Check sheet for the modelled part. Datum: model origin and axes. Units: mm. Face numbers are marked on the shaded views. A direction names the side the tool comes from. Round coordinates to 2 decimals unless told otherwise and drop trailing zeros. Order: outer loops, then holes, each group sorted by start corner. A loop starts at its lowest first (then second) coordinate and runs counter-clockwise, first axis right, second up.
(1) Mould release check, pull along X, two halves, no side actions. Record for the marked faces 1, 2 and 3: released by +X, released by -X, zero draft, split by the parting line, or undercut.
(2) Depth check by flat-ended pin: pin 1 (1.5 mm diameter, centred on x = -23.5, y = -3, fed in from +Z); pin 2 (8 mm diameter, centred on x = 11, y = -14.5, fed in from -Z); pin 3 (3 mm diameter, centred on x = -17.5, y = -14.5, fed in from -Z). Enter the tip coordinate at first touch or a pass-through.
(3) Sectioned sample at C-C, the plane y = -4. Count the separate pieces of the cut face and the enclosed holes in it, and give its area (3 significant figures).
(4) Sectioned sample at B-B, the plane y = -12.5. Enter the section's corners in (x, z).
(5) Tool access check on the marked faces 4 and 5. Record the directions out of +Z, -Z, +X, -X, +Y, -Y that give a thin tool (end or side, any length) a straight path to the whole face; none if there is none.
(6) Thickness scan on probe 1 along Z at (x, y) = (0, -0.6); probe 2 along Z at (x, y) = (0, -9.5); probe 3 along X at (y, z) = (-2, -8). Record the ranges inside material, lowest first.
(7) Sectioned sample at A-A, the plane z = 0. Enter the section's corners in (x, y).
```python
from build123d import *

# Parameters (mm, degrees)
SKETCH_R        = 29.75
PAD_DEPTH       = 19
POCKET_DEPTH    = 2
SKETCH002_R     = 5
HOLE_DEPTH      = 17.001
SKETCH003_R     = 2.5
HOLE001_DEPTH   = 17.001
POCKET001_DEPTH = 7
SKETCH005_R     = 7
POCKET002_DEPTH = 2
FILLET_R        = 0.5


with BuildPart() as part:
    # Sketch → Pad (new body)
    with BuildSketch(Plane.XZ):
        Circle(SKETCH_R)
    extrude(amount=PAD_DEPTH)

    # Sketch001 (on Face3 of Pad) → Pocket (cut)
    with BuildSketch(Plane.XZ.offset(19)):
        Polygon((-10.2, 27.94678), (-10.2, 10.2), (-27.94678, 10.2), (-38.800591, 2.809986), (-27.94678, -10.2), (-10.2, -10.2), (-10.2, -27.94678), (0.437611, -41.292454), (10.2, -27.94678), (10.2, -10.2), (27.94678, -10.2), (40.756752, -1.838068), (27.94678, 10.2), (10.2, 10.2), (10.2, 27.94678), (-0.319049, 40.318684), align=None)
    extrude(amount=-POCKET_DEPTH, mode=Mode.SUBTRACT)

    # Sketch002 (on Face3 of Pocket) → Hole (cut, through all)
    with BuildSketch(Plane.XZ.offset(17)):
        Circle(SKETCH002_R)
    extrude(amount=-HOLE_DEPTH, mode=Mode.SUBTRACT)

    # Sketch003 (on Face3 of Hole) → Hole001 (cut, through all)
    with BuildSketch(Plane.XZ.offset(17)):
        with Locations((0, 22.5)):
            Circle(SKETCH003_R)
        with Locations((22.5, 0)):
            Circle(SKETCH003_R)
        with Locations((0, -22.5)):
            Circle(SKETCH003_R)
        with Locations((-22.5, 0)):
            Circle(SKETCH003_R)
    extrude(amount=-HOLE001_DEPTH, mode=Mode.SUBTRACT)

    # Sketch004 (on Face2 of Hole001) → Pocket001 (cut)
    with BuildSketch(Plane(origin=(0, 0, 0), x_dir=(1, 0, 0), z_dir=(0, 1, 0))):
        with BuildLine():
            ThreePointArc((-21.944444, -4.96904), (-15.909903, -15.909903), (-4.96904, -21.944444))
            ThreePointArc((-3.5, -18.929286), (-4.494881, -20.310013), (-4.96904, -21.944444))
            Line((-3.5, -8.831761), (-3.5, -18.929286))
            ThreePointArc((-8.831761, -3.5), (-6.717514, -6.717514), (-3.5, -8.831761))
            Line((-18.929286, -3.5), (-8.831761, -3.5))
            ThreePointArc((-21.944444, -4.96904), (-20.310013, -4.494881), (-18.929286, -3.5))
        make_face()
        with BuildLine():
            ThreePointArc((8.831761, 3.5), (6.717514, 6.717514), (3.5, 8.831761))
            Line((3.5, 18.929286), (3.5, 8.831761))
            ThreePointArc((3.5, 18.929286), (4.494881, 20.310013), (4.96904, 21.944444))
            ThreePointArc((21.944444, 4.96904), (15.909903, 15.909903), (4.96904, 21.944444))
            ThreePointArc((21.944444, 4.96904), (20.310013, 4.494881), (18.929286, 3.5))
            Line((8.831761, 3.5), (18.929286, 3.5))
        make_face()
        with BuildLine():
            ThreePointArc((18.929286, -3.5), (20.310013, -4.494881), (21.944444, -4.96904))
            ThreePointArc((4.96904, -21.944444), (15.909903, -15.909903), (21.944444, -4.96904))
            ThreePointArc((4.96904, -21.944444), (4.494881, -20.310013), (3.5, -18.929286))
            Line((3.5, -8.831761), (3.5, -18.929286))
            ThreePointArc((3.5, -8.831761), (6.717514, -6.717514), (8.831761, -3.5))
            Line((8.831761, -3.5), (18.929286, -3.5))
        make_face()
        with BuildLine():
            Line((-3.5, 8.831761), (-3.5, 18.929286))
            ThreePointArc((-4.96904, 21.944444), (-4.494881, 20.310013), (-3.5, 18.929286))
            ThreePointArc((-4.96904, 21.944444), (-15.909903, 15.909903), (-21.944444, 4.96904))
            ThreePointArc((-18.929286, 3.5), (-20.310013, 4.494881), (-21.944444, 4.96904))
            Line((-18.929286, 3.5), (-8.831761, 3.5))
            ThreePointArc((-3.5, 8.831761), (-6.717514, 6.717514), (-8.831761, 3.5))
        make_face()
    extrude(amount=-POCKET001_DEPTH, mode=Mode.SUBTRACT)

    # Sketch005 (on Face2 of Pocket001) → Pocket002 (cut)
    with BuildSketch(Plane(origin=(0, 0, 0), x_dir=(1, 0, 0), z_dir=(0, 1, 0))):
        Circle(SKETCH005_R)
    extrude(amount=-POCKET002_DEPTH, mode=Mode.SUBTRACT)

    # Sketch006 (on DatumPlane) → Groove (revolve, cut)
    with BuildSketch(Plane(origin=(29.75, 0, 0), x_dir=(-1, 0, 0), z_dir=(0, 0, -1))):
        Polygon((0, -14), (1.5, -19), (0, -19), align=None)
    revolve(axis=Axis((0, 0, 0), (0, 1, 0)), mode=Mode.SUBTRACT)

    # Fillet
    fillet_edges = [part.edges().sort_by_distance(p)[0] for p in [
        (-29.75, 0, 0),
    ]]
    fillet(fillet_edges, radius=FILLET_R)


solid = part.part
```
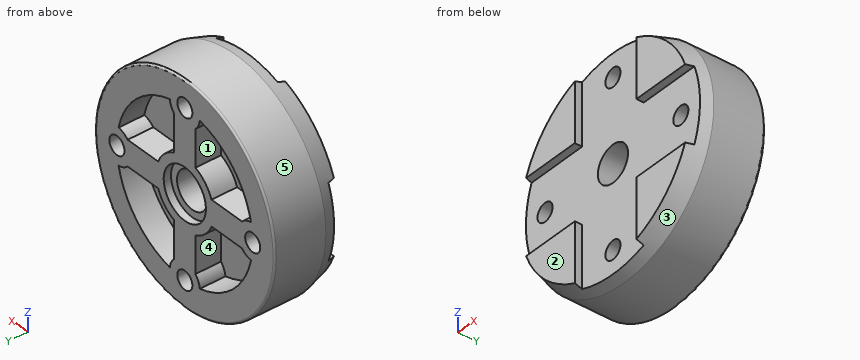
Derived:
1. face 1: undercut
1. face 2: zero draft
1. face 3: split by the parting line
2. pin 1: stops at z = 19.17
2. pin 2: stops at z = -28.91
2. pin 3: stops at z = -25.03
3. separate pieces: 1
3. enclosed holes: 9
3. area: 1,710 mm2
4. outline: circle Ø59.5 at (0, 0); hole circle Ø5 at (-22.5, 0); hole circle Ø10 at (0, 0); hole circle Ø5 at (0, -22.5); hole circle Ø5 at (0, 22.5); hole circle Ø5 at (22.5, 0)
5. face 4: +Y
5. face 5: +Y, -Y
6. probe 1: z = -29.75 to -25, -20 to -7, 7 to 20, 25 to 29.75
6. probe 2: z = -29.75 to -25, -20 to -5, 5 to 20, 25 to 29.75
6. probe 3: x = -28.65 to -21.03, -5.12 to 5.12, 21.03 to 28.65
7. outline: (-29.75, -14) - (-28.85, -17) - (-25, -17) - (-25, 0) - (-29.25, 0) arc R0.5 ccw to (-29.75, -0.5) - close; (-20, -17) - (-5, -17) - (-5, -2) - (-7, -2) - (-7, 0) - (-20, 0) - close; (5, -17) - (20, -17) - (20, 0) - (7, 0) - (7, -2) - (5, -2) - close; (25, -17) - (28.85, -17) - (29.75, -14) - (29.75, -0.5) arc R0.5 ccw to (29.25, 0) - (25, 0) - close
